Source: CAD feature listing. Evaluate the final solid. Frame: model axes, mm. A direction names the side the tool comes from. Give positions to 0.01 mm unless a question says otherwise; leave off trailing zeros. Write each loop counter-clockwise with the first axis right and the second up, starting at its lowest first coordinate (ties: lowest second). Pieces come first, ordered by that corner, then holes. Notation, with made-up numbers: (54.25, 58) -> (84.25, 58) arc R24 ccw to (84.25, 92) -> close; hole circle Ø7 at (-14, -27). An arc over 180 degrees is marked (long way). Answer as a JSON object with one key per item and string values. Group by question number.
Item 1: Ray query, probe 1 along Y at (x, z) = (25.05, 4); probe 2 along X at (y, z) = (-50.3, 4.6); probe 3 along X at (y, z) = (47.5, 4.2). Return the intervals inside material, ascending. Write a range as from..to.
Item 2: Pull-direction query (Y, two-part tool) for faces 1 (the face through (-1, 62.6, 3)), 2 (the face through (-50.2, -52.9, 4.5)), 3 (the face through (62.5, 1, 3)); classes: pulls with the +Y half, pulls with the -Y half, needs draft (parallel to the pull), parting line crosses it, or undercut.
Item 3: Access query for faces 4 (the face through (-53.606, 52.569, 1.521)), 5 (the face through (52.326, -51.287, 4.521)). Directions: +Z, -Z, +X, -X, +Y, -Y. A direction counts if a zero-diameter tool reaches every point of the face in a straight line with its end or side. Return the directions, or none.
Item 4: Section query A-A on x = 25.05. Return the cut outline in (y, z).
Item 5: First-contact query: pin 1 Ø4.5 at (x, y) = (-48, 51.5) entering from -Z; pin 2 Ø4.5 at (x, y) = (50.1, 50.53) entering from +Z. Flat tips, straight axial feed; report the tip coordinate or a pass-through.
Item 6: Section query C-C on y = -50.3. Return the cut outline in (x, z), plus the area to 3 significant figures.
Item 7: Section query B-B on y = 50.3. Return the cut outline in (x, z), plus the area to 3 significant figures.
Autodesk Inventor part; units mm, degrees
ref_plane "YZ Plane" through (0, 0, 0) normal (1, 0, 0) x (0, 1, 0)
ref_plane "XZ Plane" through (0, 0, 0) normal (0, 1, 0) x (-1, 0, 0)
ref_plane "XY Plane" through (0, 0, 0) normal (0, 0, 1) x (1, 0, 0)
ref_plane "Work Plane1" through (0, 0, 0) normal (0, 0, 1) x (1, 0, 0)
sketch "Sketch3" plane through (0, 0, 0) normal (0, 0, 1) x (1, 0, 0)
  line L0 (62.5, 62.6) -> (62.5, -62.6)
  line L1 (62.5, -62.6) -> (-62.5, -62.6)
  line L2 (62.5, 62.6) -> (62.5, -62.6)
  line L3 (-62.5, 62.6) -> (62.5, 62.6)
  line L4 (-62.5, -62.6) -> (-62.5, 62.6)
  line L5 (62.5, -62.6) -> (-62.5, -62.6)
  point P0 (0, 0)
  point P1 (50.2, -50.3)
  point P2 (25.05, -50.3)
  point P3 (-0.1, -50.3)
  point P4 (-25.25, -50.3)
  point P5 (-50.4, -50.3)
  point P6 (-50.4, 50.3)
  point P7 (-25.25, 50.3)
  point P8 (-0.1, 50.3)
  point P9 (25.05, 50.3)
  point P10 (50.2, 50.3)
extrude "Extrusion1" add sketch "Sketch3" along normal blind 6
sketch "Sketch4" plane through (0, 0, 0) normal (0, 0, -1) x (-1, 0, 0)
  point P0 (0, 0)
  point P1 (50.5386, 50.0642)
  point P2 (0.1554, 50.4302)
  point P3 (-50.0965, 50.5314)
hole "Hole1" at (50.0965, 50.5314, 0) direction (0, 0, 1) diameter 7.2 end through all counterbore diameter 12.25 counterbore depth 3
sketch "Sketch5" plane through (0, 0, 0) normal (0, 0, -1) x (-1, 0, 0)
  point P0 (0, 0)
  point P1 (-49.8367, -50.7343)
  point P2 (50.1286, -50.3518)
  point P3 (49.7277, 50.0962)
hole "Hole2" at (49.8367, -50.7343, 0) at (-50.1286, -50.3518, 0) at (-49.7277, 50.0962, 0) direction (0, 0, 1) diameter 5.1 end through all counterbore diameter 9.2 counterbore depth 3
sketch "Sketch6" plane through (0, 0, 6) normal (0, 0, 1) x (1, 0, 0)
  point P0 (0, 0)
  point P1 (-25.25, -50.3)
  point P2 (25.05, -50.3)
  point P3 (25.05, 50.3)
  point P4 (-25.25, 50.3)
hole "Hole3" at (-25.25, -50.3, 6) at (25.05, -50.3, 6) at (25.05, 50.3, 6) at (-25.25, 50.3, 6) direction (0, 0, -1) diameter 4.2 end through all
properties part number "X axis carriage small side_3DPrint"
Worked answers:
{
 "1": {"probe 1": "-62.6..-52.4, -48.2..48.2, 52.4..62.6", "probe 2": "-62.5..-52.68, -47.58..-27.35, -23.15..22.95, 27.15..47.32, 52.35..62.5", "probe 3": "-62.5..48.15, 52.04..62.5"},
 "2": {"face 1": "pulls with the +Y half", "face 2": "undercut", "face 3": "needs draft"},
 "3": {"face 4": "-Z", "face 5": "+Z, -Z"},
 "4": {"outline": "(-62.6, 0) -> (-52.4, 0) -> (-52.4, 6) -> (-62.6, 6) -> close; (-48.2, 0) -> (48.2, 0) -> (48.2, 6) -> (-48.2, 6) -> close; (52.4, 0) -> (62.6, 0) -> (62.6, 6) -> (52.4, 6) -> close"},
 "5": {"pin 1": "z = 3", "pin 2": "through"},
 "6": {"outline": "(-62.5, 0) -> (-54.73, 0) -> (-54.73, 3) -> (-52.68, 3) -> (-52.68, 6) -> (-62.5, 6) -> close; (-47.58, 3) -> (-45.53, 3) -> (-45.53, 0) -> (-27.35, 0) -> (-27.35, 6) -> (-47.58, 6) -> close; (-23.15, 0) -> (22.95, 0) -> (22.95, 6) -> (-23.15, 6) -> close; (27.15, 0) -> (45.26, 0) -> (45.26, 3) -> (47.32, 3) -> (47.32, 6) -> (27.15, 6) -> close; (52.35, 3) -> (54.42, 3) -> (54.42, 0) -> (62.5, 0) -> (62.5, 6) -> (52.35, 6) -> close", "area": "614 mm^2"},
 "7": {"outline": "(-62.5, 0) -> (-54.32, 0) -> (-54.32, 3) -> (-52.27, 3) -> (-52.27, 6) -> (-62.5, 6) -> close; (-47.19, 3) -> (-45.13, 3) -> (-45.13, 0) -> (-27.35, 0) -> (-27.35, 6) -> (-47.19, 6) -> close; (-23.15, 0) -> (22.95, 0) -> (22.95, 6) -> (-23.15, 6) -> close; (27.15, 0) -> (43.98, 0) -> (43.98, 3) -> (46.5, 3) -> (46.5, 6) -> (27.15, 6) -> close; (53.69, 3) -> (56.22, 3) -> (56.22, 0) -> (62.5, 0) -> (62.5, 6) -> (53.69, 6) -> close", "area": "598 mm^2"}
}
